```python
from build123d import *

# Parameters (mm, degrees)
BOSS_EXTRUDE1_DEPTH              = 510
CHAMFER6_SIZE                    = 50.8
CHAMFER7_SIZE                    = 50.8
BOTTOMHOLES_SKETCH3_R            = 1.5875
BOTTOMHOLES_CUT_EXTRUDE1_DEPTH   = 514.152803753
BACKSIDEHOLES_SKETCH2_R          = 1.5875
BACKSIDEHOLES_CUT_EXTRUDE2_DEPTH = 514.152803753


with BuildPart() as part:
    # Sketch1 → Boss-Extrude1 (new body)
    with BuildSketch(Plane(origin=(0, 0, 0), x_dir=(0, 0, -1), z_dir=(1, 0, 0))):
        Polygon((0, 0), (-50.8, 0), (-50.8, 3.175), (-3.175, 3.175), (-3.175, 25.4), (0, 25.4), align=None)
    extrude(amount=BOSS_EXTRUDE1_DEPTH)

    # Chamfer6
    chamfer6_edges = [part.edges().sort_by_distance(p)[0] for p in [
        (510, 1.5875, 50.8),
    ]]
    chamfer(chamfer6_edges, length=CHAMFER6_SIZE - 0.0001)  # a hair under: the kernel refuses the full size

    # Chamfer7
    chamfer7_edges = [part.edges().sort_by_distance(p)[0] for p in [
        (0, 1.5875, 50.8),
    ]]
    chamfer(chamfer7_edges, length=CHAMFER7_SIZE - 0.0001)  # a hair under: the kernel refuses the full size

    # BottomHoles-Sketch3 → BottomHoles-Cut-Extrude1 (cut, through all)
    with BuildSketch(Plane.XZ):
        with Locations(Location((39.6875, 11.1125, 0), (0, 0, 270))):
            Circle(BOTTOMHOLES_SKETCH3_R)
        with Locations(Location((470.3125, 11.1125, 0), (0, 0, 270))):
            Circle(BOTTOMHOLES_SKETCH3_R)
        with Locations(Location((127.5, 11.1125, 0), (0, 0, 270))):
            Circle(BOTTOMHOLES_SKETCH3_R)
        with Locations(Location((255, 11.1125, 0), (0, 0, 270))):
            Circle(BOTTOMHOLES_SKETCH3_R)
        with Locations(Location((382.5, 11.1125, 0), (0, 0, 270))):
            Circle(BOTTOMHOLES_SKETCH3_R)
    extrude(amount=-BOTTOMHOLES_CUT_EXTRUDE1_DEPTH, mode=Mode.SUBTRACT)

    # BackSideHoles-Sketch2 → BackSideHoles-Cut-Extrude2 (cut, through all)
    with BuildSketch(Plane(origin=(0, 0, 0), x_dir=(-1, 0, 0), z_dir=(0, 0, -1))):
        with Locations(Location((-498.8875, 17.4625, 0), (0, 0, 90))):
            Circle(BACKSIDEHOLES_SKETCH2_R)
        with Locations(Location((-489.3625, 17.4625, 0), (0, 0, 90))):
            Circle(BACKSIDEHOLES_SKETCH2_R)
        with Locations(Location((-20.6375, 17.4625, 0), (0, 0, 90))):
            Circle(BACKSIDEHOLES_SKETCH2_R)
        with Locations(Location((-11.1125, 17.4625, 0), (0, 0, 90))):
            Circle(BACKSIDEHOLES_SKETCH2_R)
        with Locations(Location((-20.6375, 11.1125, 0), (0, 0, 90))):
            Circle(BACKSIDEHOLES_SKETCH2_R)
        with Locations(Location((-489.3625, 11.1125, 0), (0, 0, 90))):
            Circle(BACKSIDEHOLES_SKETCH2_R)
        with Locations(Location((-382.5, 11.1125, 0), (0, 0, 90))):
            Circle(BACKSIDEHOLES_SKETCH2_R)
        with Locations(Location((-255, 11.1125, 0), (0, 0, 90))):
            Circle(BACKSIDEHOLES_SKETCH2_R)
        with Locations(Location((-127.5, 11.1125, 0), (0, 0, 90))):
            Circle(BACKSIDEHOLES_SKETCH2_R)
    extrude(amount=-BACKSIDEHOLES_CUT_EXTRUDE2_DEPTH, mode=Mode.SUBTRACT)


solid = part.part
```
Work out the finished part from the listing and answer in its coordinate system (mm). A direction names the side the tool comes from. Coordinates: 2 decimals unless noted, no trailing zeros. Write each loop counter-clockwise with the first axis right and the second up, starting at its lowest first coordinate (ties: lowest second). Pieces come first, ordered by that corner, then holes. Notation, with made-up numbers: (-5, 19.25) - (40, 19.25) arc R9 ccw to (40, 35.25) - close; hole circle Ø1 at (7, -16.5). An arc over 180 degrees is marked (long way). Answer as a JSON object with one key per item and string values.
Q1. Find section A-A (x = 345). Write down the section's boundary in (y, z) (3 decimals), plus the area to 3 significant figures.
Results list:
{"outline": "(0, 0) - (25.4, 0) - (25.4, 3.175) - (3.175, 3.175) - (3.175, 50.8) - (0, 50.8) - close", "area": "232 mm^2"}
Q2. Given pin 1 Ø24 at (x, z) = (319, 34) entering from +Y (3 decimals); pin 2 Ø4 at (x, y) = (20.64, 17.46) entering from +Z (3 decimals), each flat-ended and moving along its own axis, determine where each tip first touches the part or whether it passes through.
Results list:
{"pin 1": "stops at y = 3.175", "pin 2": "stops at z = 3.175"}
Q3. Find section C-C (z = 23). Write down the section's boundary in (x, y) (3 decimals), plus the area to 3 significant figures.
Results list:
{"outline": "(23, 0) - (487, 0) - (487, 3.175) - (23, 3.175) - close", "area": "1,470 mm^2"}
Q4. Find section B-B (z = 46). Write down the section's boundary in (x, y) (3 decimals).
Results list:
{"outline": "(46, 0) - (464, 0) - (464, 3.175) - (46, 3.175) - close"}
Q5. Which of the six approach directions +Z, -Z, +X, -X, +Y, -Y give full straight-line access (tool end or side, diameter ignored) to faces 1 (the flat face through (251, 13, 0)), 2 (the flat face through (251, 3.175, 27))?
Results list:
{"face 1": "-Z, +X, -X, +Y, -Y", "face 2": "+Z, +X, -X, +Y"}
Q6. Consider L1, parallel to Z at x = 255, y = 1.85 (3 decimals); L2, parallel to Y at x = 255, z = 1 (3 decimals); L3, parallel to Z at x = 486, y = 11 (3 decimals). Determine where each line is inside the solid, lowest interval first. Write a range as from..to.
Results list:
{"L1": "z = 0..9.525, 12.7..50.8", "L2": "y = 0..9.525, 12.7..25.4", "L3": "z = 0..3.175"}
